Autodesk Inventor part; units mm, degrees
ref_plane "YZ Plane" through (0, 0, 0) normal (1, 0, 0) x (0, 1, 0)
ref_plane "XZ Plane" through (0, 0, 0) normal (0, 1, 0) x (-1, 0, 0)
ref_plane "XY Plane" through (0, 0, 0) normal (0, 0, 1) x (1, 0, 0)
sketch "Sketch1" plane through (0, 0, 0) normal (0, 0, 1) x (1, 0, 0)
  line L0 (-17.78, 0) -> (17.78, 0)
  line L1 (0, -17.78) -> (0, 17.78)
  circle A0 centre (0, 0) radius 12.7
  circle A1 centre (0, 0) radius 4.7625
  dimension "d0" = 9.525
  dimension "d1" = 25.4
extrude "Base" add sketch "Sketch1" along normal mid plane 7.1425 contours A1 L1 A0 L0 | L0 A0 L1 A1 | A1 L0 A0 L1 | L1 A0 L0 A1
sketch "Sketch2" plane through (0, 0, 3.5712) normal (0, 0, 1) x (1, 0, 0)
  circle A0 centre (0, 0) radius 12.7
  circle A1 centre (0, 0) radius 11.1125
  dimension "d4" = 22.225
extrude "Flange Cutaway" cut sketch "Sketch2" against normal blind 5.5677
sketch "Sketch3" plane through (0, 0, 3.5712) normal (0, 0, 1) x (1, 0, 0)
  circle A0 centre (0, 0) radius 11.1125
  circle A1 centre (0, 0) radius 4.7625
  circle A2 centre (0, 0) radius 6.35
  circle A3 centre (0, 0) radius 8.7312
  dimension "d7" = 1.5875
  dimension "d8" = 2.3813
extrude "Cutaway" cut sketch "Sketch3" against normal blind 0.3969 contours A3
mirror "Mirror1" about plane through (0, 0, 0) normal (0, 0, 1) of "Cutaway"
properties part number "bearing_1.125OD" material "Steel"
Model file for the job. Use its own axes, mm. A direction names the side the tool comes from. Give positions to 0.01 mm unless a question says otherwise; leave off trailing zeros. Order: outer loops, then holes, each group sorted by start corner. A loop starts at its lowest first (then second) coordinate and runs counter-clockwise, first axis right, second up. Notation, with made-up numbers: M 25.5,70.5 L 29.5,70.5 A26 cw 29.5,100.5 Z; hole C 31,8 d4. An arc over 180 degrees is marked long. Write item = value, one per line.
Q1. Two-plate mould, pull along X, no slides. Class faces 1 (the cylindrical face through (10.6, 3.34, 0.83)), 2 (the cylindrical face through (-1.38, -6.2, 3.38)), 3 (the flat face through (1, 5, -3.571)): pulls with the +X half, pulls with the -X half, needs draft (parallel to the pull), parting line crosses it, or undercut.
Derived:
face_1 = parting line crosses it
face_2 = undercut
face_3 = needs draft
Q2. Cut at A-A, the plane y = 0. List the corners of the cut face in (x, z).
Derived:
outline = M -12.7,-3.57 L -8.73,-3.57 L -8.73,-3.17 L -6.35,-3.17 L -6.35,-3.57 L -4.76,-3.57 L -4.76,3.57 L -6.35,3.57 L -6.35,3.17 L -8.73,3.17 L -8.73,3.57 L -11.11,3.57 L -11.11,-2 L -12.7,-2 Z; M 4.76,-3.57 L 6.35,-3.57 L 6.35,-3.17 L 8.73,-3.17 L 8.73,-3.57 L 12.7,-3.57 L 12.7,-2 L 11.11,-2 L 11.11,3.57 L 8.73,3.57 L 8.73,3.17 L 6.35,3.17 L 6.35,3.57 L 4.76,3.57 Z
Q3. Flat gauge pins, fed straight in: pin 1 (1 mm diameter, centred on x = -2, z = 0, fed in from +Y); pin 2 (1.5 mm diameter, centred on x = 5.5, z = -2, fed in from -Y); pin 3 (3 mm diameter, centred on y = 4.5, z = -2, fed in from -X). Where does each tip first touch, or does it go through?
Derived:
pin_1 = 11.01
pin_2 = -11.78
pin_3 = -12.34
Q4. Cut at C-C, the plane z = -1.5. List the corners of the cut face in (x, y) (1 decimal).
Derived:
outline = C 0,0 d22.2; hole C 0,0 d9.5
Q5. Tool access for faces 4 (the flat face through (3, 9, -3.571)), 5 (the cylindrical face through (-1.137, -8.657, -3.376)), 6 (the flat face through (0.88, -11.23, -1.996)): list every direction of +Z, -Z, +X, -X, +Y, -Y with a clear straight run to the whole face (end or side of a thin tool).
Derived:
face_4 = -Z, +X, -X, +Y, -Y
face_5 = -Z
face_6 = +Z
Q6. Drill centre lines: line 1 (Y direction, x = 0, z = 3.4); line 2 (Y direction, x = 0, z = 1.75); line 3 (Y direction, x = 0, z = -3.3). Where is each one in solid material? Low to high. Write a range as [from, to].
Derived:
line_1 = [-11.11, -8.73], [-6.35, -4.76], [4.76, 6.35], [8.73, 11.11]
line_2 = [-11.11, -4.76], [4.76, 11.11]
line_3 = [-12.7, -8.73], [-6.35, -4.76], [4.76, 6.35], [8.73, 12.7]
Q7. Cut at D-D, the plane x = 7. List the corners of the cut face in (y, z), then the cut area to 3 significant figures.
Derived:
outline = M -10.6,-3.57 L -5.22,-3.57 L -5.22,-3.17 L 5.22,-3.17 L 5.22,-3.57 L 10.6,-3.57 L 10.6,-2 L 8.63,-2 L 8.63,3.57 L 5.22,3.57 L 5.22,3.17 L -5.22,3.17 L -5.22,3.57 L -8.63,3.57 L -8.63,-2 L -10.6,-2 Z
area = 121 mm2
